from build123d import *

# Parameters (mm, degrees)
F0_R     = 3.7
F1_DEPTH = 13.5
F2_R     = 5.08
F4_D     = 3.81


with BuildPart() as f1:
    # F0 (on Top) → F1 (new body, symmetric)
    with BuildSketch(Plane.XY):
        with BuildLine():
            Line((47.9, 2.3014477862), (47.9, 7.887150161))
            ThreePointArc((47.9, 7.887150161), (44.2, 4.187150161), (40.5, 7.887150161))
            Line((40.5, 7.887150161), (40.5, 2.3014477862))
            ThreePointArc((40.5, 2.3014477862), (40.7473700627, 2.1452499933), (41.0013230857, 2))
            Line((41.0013230857, 2), (47.3986769143, 2))
            ThreePointArc((47.3986769143, 2), (47.6526299373, 2.1452499933), (47.9, 2.3014477862))
        make_face()
        with BuildLine():
            ThreePointArc((40.5, 7.887150161), (44.2, 11.587150161), (47.9, 7.887150161))
            Line((47.9, 7.887150161), (47.9, 2.3014477862))
            ThreePointArc((47.9, 2.3014477862), (50.1025456639, 4.7169726099), (50.9000053, 7.887150161))
            ThreePointArc((50.9000053, 7.887150161), (44.2, 14.587155461), (37.4999947, 7.887150161))
            ThreePointArc((37.4999947, 7.887150161), (38.2974543361, 4.7169726099), (40.5, 2.3014477862))
            Line((40.5, 2.3014477862), (40.5, 7.887150161))
        make_face()
        with BuildLine():
            ThreePointArc((50.9000053, 7.887150161), (50.1025456639, 4.7169726099), (47.9, 2.3014477862))
            Line((47.9, 2.3014477862), (47.9, 2))
            Line((47.9, 2), (47.9, -2))
            Line((47.9, -2), (50.9000053, -2))
            Line((50.9000053, -2), (50.9000053, 7.887150161))
        make_face()
        with BuildLine():
            Line((40.5, 2), (40.5, 2.3014477862))
            ThreePointArc((40.5, 2.3014477862), (38.2974543361, 4.7169726099), (37.4999947, 7.887150161))
            Line((37.4999947, 7.887150161), (37.4999947, 2))
            Line((37.4999947, 2), (40.5, 2))
        make_face()
        with BuildLine():
            Line((47.9, -2), (47.9, 2))
            Line((47.9, 2), (47.3986769143, 2))
            ThreePointArc((47.3986769143, 2), (44.2, 1.187144861), (41.0013230857, 2))
            Line((41.0013230857, 2), (40.5, 2))
            Line((40.5, 2), (37.4999947, 2))
            Line((37.4999947, 2), (0, 2))
            Line((0, 2), (0, -2))
            Line((0, -2), (47.9, -2))
        make_face()
        with BuildLine():
            ThreePointArc((41.0013230857, 2), (44.2, 1.187144861), (47.3986769143, 2))
            Line((47.3986769143, 2), (41.0013230857, 2))
        make_face()
        with BuildLine():
            Line((-47.9, -2), (0, -2))
            Line((0, -2), (0, 2))
            Line((0, 2), (-37.4999947, 2))
            Line((-37.4999947, 2), (-41.0013230857, 2))
            ThreePointArc((-41.0013230857, 2), (-44.2, 1.187144861), (-47.3986769143, 2))
            ThreePointArc((-47.3986769143, 2), (-49.958525128, 4.4623203301), (-50.9000053, 7.887150161))
            Line((-50.9000053, 7.887150161), (-50.9000053, -2))
            Line((-50.9000053, -2), (-47.9, -2))
        make_face()
        with BuildLine():
            Line((-41.0013230857, 2), (-37.4999947, 2))
            Line((-37.4999947, 2), (-37.4999947, 7.887150161))
            ThreePointArc((-37.4999947, 7.887150161), (-38.441474872, 4.4623203301), (-41.0013230857, 2))
        make_face()
        with BuildLine():
            ThreePointArc((-47.3986769143, 2), (-44.2, 1.187144861), (-41.0013230857, 2))
            Line((-41.0013230857, 2), (-47.3986769143, 2))
        make_face()
        with BuildLine():
            Line((-47.3986769143, 2), (-41.0013230857, 2))
            ThreePointArc((-41.0013230857, 2), (-38.441474872, 4.4623203301), (-37.4999947, 7.887150161))
            ThreePointArc((-37.4999947, 7.887150161), (-44.2, 14.587155461), (-50.9000053, 7.887150161))
            ThreePointArc((-50.9000053, 7.887150161), (-49.958525128, 4.4623203301), (-47.3986769143, 2))
        make_face()
        with Locations((-44.2, 7.887150161)):
            Circle(F0_R, mode=Mode.SUBTRACT)
    extrude(amount=F1_DEPTH, both=True)

    # F2
    f2_edges = [f1.edges().sort_by_distance(p)[0] for p in [
        (50.900005, -2, 0),
        (-50.900005, -2, 0),
    ]]
    fillet(f2_edges, radius=F2_R)

    # F4 (through all)
    with Locations(Plane.XZ.offset(2)):
        with Locations((-30.41523, 9.59459), (-30.41523, -9.59459), (30.41523, -9.59459), (30.41523, 9.59459)):
            Hole(F4_D / 2)


solid = f1.part
Source: CAD feature listing. Evaluate the final solid. Frame: model axes, mm. A direction names the side the tool comes from. Round coordinates to 2 decimals unless told otherwise and drop trailing zeros. Loops run counter-clockwise (first coordinate to the right, second up) from the corner with the lowest first, then second, coordinate; pieces in that order, holes last. Notation, with made-up numbers: (58, 73) -> (83, 73) arc R17 ccw to (83, 83) -> close; hole circle Ø1 at (-0.5, -23). An arc over 180 degrees is marked (long way). Answer as a JSON object with one key per item and string values. Group by question number.
Q1. Ray query, line 1 (X direction, y = 7.75, z = -3); line 2 (X direction, y = 3.25, z = -7.5); line 3 (X direction, y = 10, z = -2.5). Return the intervals inside material, ascending. Write a range as from..to.
Q2. Contact query for flat-ended pins moving along their axis: P1, Ø3, axis at y = 11.5, z = -0.5, coming from the +X side; P2, Ø1, axis at y = 10.5, z = -9.5, coming from the -X side; P3, Ø8.5, axis at x = -44.2, y = 7.89, coming from the -Z side; P4, Ø5, axis at x = -30.42, z = -9.59, coming from the +Y side. Output: stop coordinate, or through.
Q3. Section query A-A (x = 44.2). Output: boundary loops of the cut face in (y, z).
Q4. Section query B-B (x = 29.5). Output: boundary loops of the cut face in (y, z).
Q5. Section query D-D (x = -27.5). Output: boundary loops of the cut face in (y, z).
Q6. Access query for faces 4 (the flat face through (-50.9, 6, 0)), 5 (the flat face through (37.5, 5, 0)). Directions: +Z, -Z, +X, -X, +Y, -Y. A direction counts if a zero-diameter tool reaches every point of the face in a straight line with its end or side. Return the directions, or none.
Q7. Section query C-C (y = -0.75). Output: boundary loops of the cut face in (x, z) (3 decimals), plus the area to 3 significant figures.
Q8. Mould query, pull axis X, two halves, no side actions, for faces 1 (the cylindrical face through (49.451, -0.472, -0.189)), 2 (the flat face through (-4, 0, 13.5)), 3 (the cylindrical face through (28.6, 0.03, -9.02)). Classes: pulls with the +X half, pulls with the -X half, needs draft (parallel to the pull), parting line crosses it, or undercut.
Completed:
{
 "1": {"line 1": "-50.9..-47.9, -40.5..-37.5, 37.5..40.5, 47.9..50.9", "line 2": "-50.9..-37.5, 37.5..50.9", "line 3": "-50.56..-47.24, -41.16..-37.84, 37.84..41.16, 47.24..50.56"},
 "2": {"P1": "x = 50.56", "P2": "x = -50.56", "P3": "z = -13.5", "P4": "y = 2"},
 "3": {"outline": "(-2, -13.5) -> (4.19, -13.5) -> (4.19, 13.5) -> (-2, 13.5) -> close; (11.59, -13.5) -> (14.59, -13.5) -> (14.59, 13.5) -> (11.59, 13.5) -> close"},
 "4": {"outline": "(-2, -13.5) -> (2, -13.5) -> (2, -11.27) -> (-2, -11.27) -> close; (-2, -7.92) -> (2, -7.92) -> (2, 7.92) -> (-2, 7.92) -> close; (-2, 11.27) -> (2, 11.27) -> (2, 13.5) -> (-2, 13.5) -> close"},
 "5": {"outline": "(-2, -13.5) -> (2, -13.5) -> (2, 13.5) -> (-2, 13.5) -> close"},
 "6": {"face 4": "+Z, -Z, -X, +Y, -Y", "face 5": "+Z, -Z, +Y"},
 "7": {"outline": "(-49.157, -13.5) -> (49.157, -13.5) -> (49.157, 13.5) -> (-49.157, 13.5) -> close; hole circle Ø3.81 at (-30.415, -9.595); hole circle Ø3.81 at (-30.415, 9.595); hole circle Ø3.81 at (30.415, -9.595); hole circle Ø3.81 at (30.415, 9.595)", "area": "2,610 mm²"},
 "8": {"face 1": "pulls with the +X half", "face 2": "needs draft", "face 3": "undercut"}
}
